Verification items for the finished model (mm, model axes). A direction names the side the tool comes from. Round coordinates to 2 decimals unless told otherwise and drop trailing zeros. Write each loop counter-clockwise with the first axis right and the second up, starting at its lowest first coordinate (ties: lowest second). Pieces come first, ordered by that corner, then holes. Notation, with made-up numbers: (45, -3.75) - (76, -3.75) arc R33 cw to (76, 25.25) - close; hole circle Ø7 at (31.25, 64). An arc over 180 degrees is marked (long way). Answer as a JSON object with one key per item and string values. Group by question number.
1) Go/stop test with flat-tipped pins: pin 1 Ø2.5 at (y, z) = (18, 23) entering from -X; pin 2 Ø1.6 at (x, z) = (-10.5, -14) entering from +Y; pin 3 Ø4 at (x, y) = (16, 7.5) entering from -Z. Record where each tip stops, or that it passes through.
2) Section check B-B (z = 9). Enter the section's corners in (x, y), then the cut area to 3 significant figures.
3) Section check A-A (y = 17.25). Enter the section's corners in (x, z), then the cut area to 3 significant figures.
4) Mould release check, pull along Z, two halves, no side actions. Record for faces 1 (the flat face through (0, 10, 30)), 2 (the flat face through (2.5, 17.5, 25.1)), 3 (the cylindrical face through (-13.157, 19.014, 26.406)): +Z half, -Z half, draft (parallel to the pull), parting line (faces both ways), or undercut.
5) Set-up check for faces 4 (the flat face through (-17, 10, -23)), 5 (the cylindrical face through (19.65, 9.86, -26.99)), 6 (the flat face through (0, 15, 25)): record each of +Z, -Z, +X, -X, +Y, -Y from which the full face is reachable in a straight line by a thin tool's end or side.
6) Section check D-D (z = 22.5). Enter the section's corners in (x, y), then the cut area to 3 significant figures.
7) Section check C-C (x = -1.5). Enter the section's corners in (y, z), then the cut area to 3 significant figures.
8) Thickness scan on line 1 (Z direction, x = 17.5, y = 17); line 2 (X direction, y = 16, z = -22.5); line 3 (Z direction, x = -17, y = 11.5). Record the ranges inside material, lowest first.
```python
from build123d import *

# Parameters (mm, degrees)
BOSS_EXTRU_1_DEPTH      = 10
ESQUISSE2_W             = 30
ESQUISSE2_H             = 40
BOSS_EXTRU_2_DEPTH      = 10
ESQUISSE3_R             = 1
BOSS_EXTRU_3_DEPTH      = 4
ESQUISSE4_W             = 5
ESQUISSE4_H             = 10
ENL_V_MAT_EXTRU_1_DEPTH = 5
ESQUISSE5_R             = 2.25
ENL_V_MAT_EXTRU_2_DEPTH = 10
CUT_EXTRUDE1_DEPTH      = 2


with BuildPart() as part:
    # Esquisse1 → Boss.-Extru.1 (new body)
    with BuildSketch(Plane(origin=(0, 0, 0), x_dir=(1, 0, 0), z_dir=(0, 1, 0))):
        with BuildLine():
            Line((-12.5, 30), (12.5, 30))
            ThreePointArc((12.5, 30), (19.571067812, 27.071067812), (22.5, 20))
            Line((22.5, 20), (22.5, -20))
            ThreePointArc((22.5, -20), (19.571067812, -27.071067812), (12.5, -30))
            Line((12.5, -30), (-12.5, -30))
            ThreePointArc((-12.5, -30), (-19.571067812, -27.071067812), (-22.5, -20))
            Line((-22.5, -20), (-22.5, 20))
            ThreePointArc((-22.5, 20), (-19.571067812, 27.071067812), (-12.5, 30))
        make_face()
    extrude(amount=BOSS_EXTRU_1_DEPTH)

    # Esquisse2 → Boss.-Extru.2 (add)
    with BuildSketch(Plane(origin=(0, 10, 0), x_dir=(1, 0, 0), z_dir=(0, 1, 0))):
        with BuildLine():
            ThreePointArc((22.5, 20), (19.571067812, 27.071067812), (12.5, 30))
            Line((12.5, 30), (-12.5, 30))
            ThreePointArc((-12.5, 30), (-19.571067812, 27.071067812), (-22.5, 20))
            Line((-22.5, 20), (-22.5, -20))
            ThreePointArc((-22.5, -20), (-19.571067812, -27.071067812), (-12.5, -30))
            Line((-12.5, -30), (12.5, -30))
            ThreePointArc((12.5, -30), (19.571067812, -27.071067812), (22.5, -20))
            Line((22.5, -20), (22.5, 20))
        make_face()
        Rectangle(ESQUISSE2_W, ESQUISSE2_H, mode=Mode.SUBTRACT)
    extrude(amount=BOSS_EXTRU_2_DEPTH)

    # Esquisse3 → Boss.-Extru.3 (add)
    with BuildSketch(Plane(origin=(0, 10, 0), x_dir=(1, 0, 0), z_dir=(0, 1, 0))):
        with Locations(Location((-10.16, 14.478, 0), (0, 0, 270))):
            Circle(ESQUISSE3_R)
        with Locations(Location((10.16, 14.478, 0), (0, 0, 270))):
            Circle(ESQUISSE3_R)
    extrude(amount=BOSS_EXTRU_3_DEPTH)

    # Esquisse4 → Enlèv. mat.-Extru.1 (cut)
    with BuildSketch(Plane(origin=(0, 20, 0), x_dir=(1, 0, 0), z_dir=(0, 1, 0))):
        with Locations((0, -25)):
            Rectangle(ESQUISSE4_W, ESQUISSE4_H)
    extrude(amount=-ENL_V_MAT_EXTRU_1_DEPTH, mode=Mode.SUBTRACT)

    # Esquisse5 → Enlèv. mat.-Extru.2 (cut)
    with BuildSketch(Plane(origin=(0, 20, 0), x_dir=(1, 0, 0), z_dir=(0, 1, 0))):
        with Locations(Location((-17.5, -22.5, 0), (0, 0, 270))):
            Circle(ESQUISSE5_R)
        with Locations(Location((17.5, -22.5, 0), (0, 0, 270))):
            Circle(ESQUISSE5_R)
        with Locations(Location((17.5, 22.5, 0), (0, 0, 270))):
            Circle(ESQUISSE5_R)
        with Locations(Location((-17.5, 22.5, 0), (0, 0, 270))):
            Circle(ESQUISSE5_R)
    extrude(amount=-ENL_V_MAT_EXTRU_2_DEPTH, mode=Mode.SUBTRACT)

    # Sketch1 → Cut-Extrude1 (cut)
    with BuildSketch(Plane(origin=(0, 20, 0), x_dir=(1, 0, 0), z_dir=(0, 1, 0))):
        with BuildLine():
            Line((-9.571067812, 27.071067812), (9.571067812, 27.071067812))
            ThreePointArc((9.571067812, 27.071067812), (13.20533493, 26.387295724), (16.342599965, 24.429488315))
            ThreePointArc((16.342599965, 24.429488315), (15.643481423, 21.228843529), (18.880326672, 20.723149337))
            ThreePointArc((18.880326672, 20.723149337), (19.396865199, 18.929482646), (19.571067812, 17.071067812))
            Line((19.571067812, 17.071067812), (19.571067812, -17.071067812))
            ThreePointArc((19.571067812, -17.071067812), (19.396865199, -18.929482646), (18.880326672, -20.723149337))
            ThreePointArc((18.880326672, -20.723149337), (15.643481423, -21.228843529), (16.342599965, -24.429488315))
            ThreePointArc((16.342599965, -24.429488315), (13.20533493, -26.387295724), (9.571067812, -27.071067812))
            Line((9.571067812, -27.071067812), (-9.571067812, -27.071067812))
            ThreePointArc((-9.571067812, -27.071067812), (-13.20533493, -26.387295724), (-16.342599965, -24.429488315))
            ThreePointArc((-16.342599965, -24.429488315), (-15.643481423, -21.228843529), (-18.880326672, -20.723149337))
            ThreePointArc((-18.880326672, -20.723149337), (-19.396865199, -18.929482646), (-19.571067812, -17.071067812))
            Line((-19.571067812, -17.071067812), (-19.571067812, 17.071067812))
            ThreePointArc((-19.571067812, 17.071067812), (-19.396865199, 18.929482646), (-18.880326672, 20.723149337))
            ThreePointArc((-18.880326672, 20.723149337), (-15.643481423, 21.228843529), (-16.342599965, 24.429488315))
            ThreePointArc((-16.342599965, 24.429488315), (-13.20533493, 26.387295724), (-9.571067812, 27.071067812))
        make_face()
        with BuildLine():
            Line((-7.571067812, 25.071067812), (7.571067812, 25.071067812))
            ThreePointArc((7.571067812, 25.071067812), (14.642135624, 22.142135624), (17.571067812, 15.071067812))
            Line((17.571067812, 15.071067812), (17.571067812, -15.071067812))
            ThreePointArc((17.571067812, -15.071067812), (14.642135624, -22.142135624), (7.571067812, -25.071067812))
            Line((7.571067812, -25.071067812), (-7.571067812, -25.071067812))
            ThreePointArc((-7.571067812, -25.071067812), (-14.642135624, -22.142135624), (-17.571067812, -15.071067812))
            Line((-17.571067812, -15.071067812), (-17.571067812, 15.071067812))
            ThreePointArc((-17.571067812, 15.071067812), (-14.642135624, 22.142135624), (-7.571067812, 25.071067812))
        make_face(mode=Mode.SUBTRACT)
    extrude(amount=-CUT_EXTRUDE1_DEPTH, mode=Mode.SUBTRACT)


solid = part.part
```
Returned:
{
 "1": {"pin 1": "x = -22.35", "pin 2": "y = 14", "pin 3": "z = -29.89"},
 "2": {"outline": "(-22.5, 0) - (22.5, 0) - (22.5, 20) - (19.57, 20) - (19.57, 18) - (17.57, 18) - (17.57, 20) - (15, 20) - (15, 10) - (-15, 10) - (-15, 20) - (-17.57, 20) - (-17.57, 18) - (-19.57, 18) - (-19.57, 20) - (-22.5, 20) - close", "area": "592 mm2"},
 "3": {"outline": "(-22.5, -20) arc R10 ccw to (-12.5, -30) - (12.5, -30) arc R10 ccw to (22.5, -20) - (22.5, 20) arc R10 ccw to (12.5, 30) - (2.5, 30) - (2.5, 20) - (15, 20) - (15, -20) - (-15, -20) - (-15, 20) - (-2.5, 20) - (-2.5, 30) - (-12.5, 30) arc R10 ccw to (-22.5, 20) - close; hole circle Ø4.5 at (-17.5, -22.5); hole circle Ø4.5 at (-17.5, 22.5); hole circle Ø4.5 at (17.5, -22.5); hole circle Ø4.5 at (17.5, 22.5)", "area": "1,300 mm2"},
 "4": {"face 1": "+Z half", "face 2": "draft", "face 3": "undercut"},
 "5": {"face 4": "+Y", "face 5": "-Z, +X, +Y, -Y", "face 6": "+Z, +Y"},
 "6": {"outline": "(-22.18, 0) - (22.18, 0) - (22.18, 20) - (19.75, 20) - (19.75, 10) - (15.25, 10) - (15.25, 18) - (14.27, 18) - (14.27, 20) - (2.5, 20) - (2.5, 15) - (-2.5, 15) - (-2.5, 20) - (-14.27, 20) - (-14.27, 18) - (-15.25, 18) - (-15.25, 10) - (-19.75, 10) - (-19.75, 20) - (-22.18, 20) - close", "area": "768 mm2"},
 "7": {"outline": "(0, -30) - (20, -30) - (20, -27.07) - (18, -27.07) - (18, -25.07) - (20, -25.07) - (20, -20) - (10, -20) - (10, 20) - (15, 20) - (15, 30) - (0, 30) - close", "area": "746 mm2"},
 "8": {"line 1": "-28.66 to -24.75, -20.25 to 20.25, 24.75 to 28.66", "line 2": "-22.18 to -19.75, -15.25 to 15.25, 19.75 to 22.18", "line 3": "-28.93 to -24.69, -20.31 to 20.31, 24.69 to 28.93"}
}
